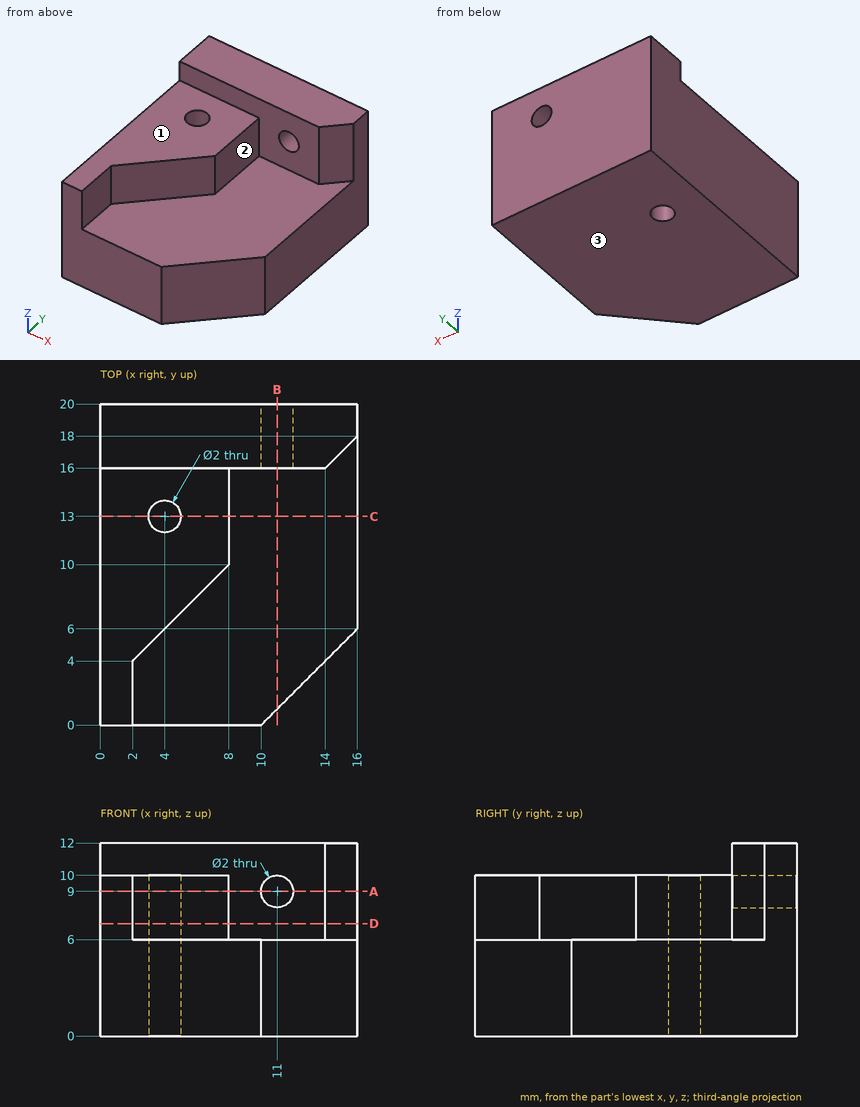
Could you check a few things on this drawing? It's one solid part, dimensions in mm from its lowest x, y, z. A direction names the side the tool comes from. Round coordinates to 2 decimals unless told otherwise and drop trailing zeros. Order: outer loops, then holes, each group sorted by start corner. A loop starts at its lowest first (then second) coordinate and runs counter-clockwise, first axis right, second up. Notation, with made-up numbers: M -15.75,21.25 L 42.25,21.25 A23 cw 42.25,39.25 Z; hole C 40.5,12.5 d2. An arc over 180 degrees is marked long. Use a Markdown table: item, result.
1) I'm going to push flat-ended pins straight in: P1, Ø4.5, axis at y = 2.5, z = 8.5, coming from the +X side; P2, Ø1.8, axis at x = 5.5, z = 9, coming from the -Y side; P3, Ø6, axis at x = 5.5, z = 7, coming from the -Y side; P4, Ø1.2, axis at y = 13.5, z = 7.5, coming from the +X side. Where does each tip first touch, or does it pass through?
Geometry says:
| item | result |
|---|---|
| P1 | stops at x = 2.75 |
| P2 | stops at y = 6.6 |
| P3 | stops at y = 0 |
| P4 | stops at x = 8 |
2) Imagine slicing it at A-A (z = 9). List the corners of the cut face in (x, y) for me, then the cut area to 3 significant figures.
Geometry says:
| item | result |
|---|---|
| outline | M 0,0 L 2,0 L 2,4 L 8,10 L 8,16 L 10,16 L 10,20 L 0,20 Z; M 12,16 L 14,16 L 16,18 L 16,20 L 12,20 Z; hole C 4,13 d2 |
| area | 137 mm² |
3) Imagine slicing it at B-B (x = 11). List the corners of the cut face in (y, z) for me, then the cut area to 3 significant figures.
Geometry says:
| item | result |
|---|---|
| outline | M 1,0 L 20,0 L 20,8 L 16,8 L 16,6 L 1,6 Z; M 16,10 L 20,10 L 20,12 L 16,12 Z |
| area | 130 mm² |
4) On a 3-axis mill with a long thin cutter (end or side, diameter ignored), from which of +Z, -Z, +X, -X, +Y, -Y can I reach the whole of each face in a straight line? I mean the marked faces 1, 2 and 3. Say none if no direction works.
Geometry says:
| item | result |
|---|---|
| face 1 | +Z, +X, -X, -Y |
| face 2 | +Z, +X, -Y |
| face 3 | -Z, +X, -X, +Y, -Y |
5) Imagine slicing it at D-D (z = 7). List the corners of the cut face in (x, y) for me.
Geometry says:
| item | result |
|---|---|
| outline | M 0,0 L 2,0 L 2,4 L 8,10 L 8,16 L 14,16 L 16,18 L 16,20 L 0,20 Z; hole C 4,13 d2 |
6) Imagine slicing it at C-C (y = 13). List the corners of the cut face in (x, z) for me, then the cut area to 3 significant figures.
Geometry says:
| item | result |
|---|---|
| outline | M 0,0 L 3,0 L 3,10 L 0,10 Z; M 5,0 L 16,0 L 16,6 L 8,6 L 8,10 L 5,10 Z |
| area | 108 mm² |
7) If I drill on line 1 along Y through (x, z) = (4, 4.25); line 2 along X through (y, z) = (19, 9); line 3 along X through (y, z) = (13, 2.75), over which ranges is the centre line in solid material (lowest first)?
Geometry says:
| item | result |
|---|---|
| line 1 | y = 0 to 12, 14 to 20 |
| line 2 | x = 0 to 10, 12 to 16 |
| line 3 | x = 0 to 3, 5 to 16 |
